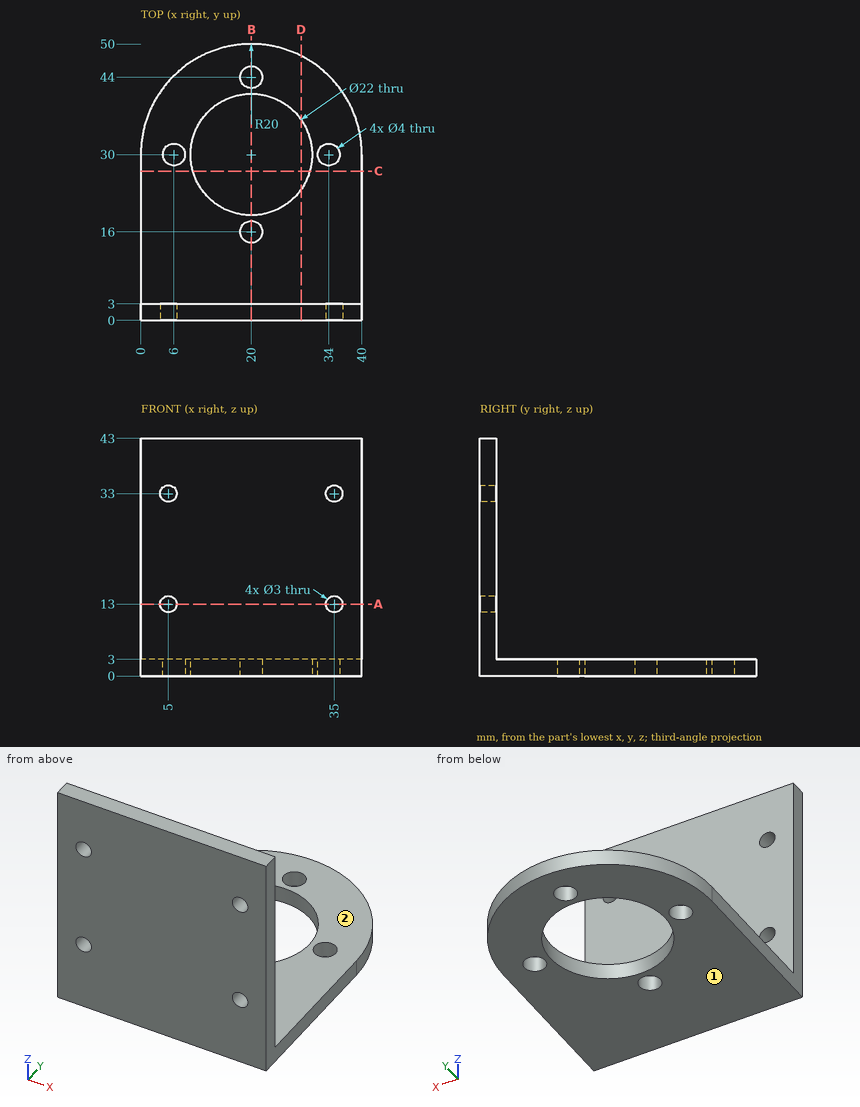
Print and shaded views of the part. All mm, measured from the part's lowest x, y and z. A direction names the side the tool comes from. Coordinates: 2 decimals unless noted, no trailing zeros. Loops run counter-clockwise (first coordinate to the right, second up) from the corner with the lowest first, then second, coordinate; pieces in that order, holes last. Notation, with made-up numbers: (74, -20.75) -> (130, -20.75) arc R24 cw to (130, 10.25) -> close; hole circle Ø11 at (-12.5, 25). An arc over 180 degrees is marked (long way). Use one line per item in the form item = value. Start each with the question number.
(1) Flat gauge pins, fed straight in: pin 1 (10 mm diameter, centred on x = 30, z = 15.5, fed in from +Y); pin 2 (20 mm diameter, centred on x = 25, y = 19.5, fed in from +Z). Where does each tip first touch, or does it go through?
(2) Probe probe 1 along Z at (x, y) = (3.5, 19.5); probe 2 along Y at (x, z) = (34, 2.2). List the from-to ranges inside material, lowest first. Write a range as from..to.
(3) Tool access for the marked faces 1 and 2: list every direction of +Z, -Z, +X, -X, +Y, -Y with a clear straight run to the whole face (end or side of a thin tool).
(4) Cut at A-A on z = 13. Give the cut face in (x, y), and give its area (3 significant figures).
(5) Cut at D-D on x = 29. Give the cut face in (y, z).
(6) Cut at C-C on y = 27. Give the cut face in (x, z).
(7) Cut at B-B on x = 20. Give the cut face in (y, z), and give its area (3 significant figures).
Values:
q1.pin_1 = 3
q1.pin_2 = 3
q2.probe_1 = 0..3
q2.probe_2 = 0..28, 32..44.28
q3.face_1 = -Z, +X, -X, +Y, -Y
q3.face_2 = +Z, +X, -X, +Y
q4.outline = (0, 0) -> (3.5, 0) -> (3.5, 3) -> (0, 3) -> close; (6.5, 0) -> (33.5, 0) -> (33.5, 3) -> (6.5, 3) -> close; (36.5, 0) -> (40, 0) -> (40, 3) -> (36.5, 3) -> close
q4.area = 102 mm2
q5.outline = (0, 0) -> (23.68, 0) -> (23.68, 3) -> (3, 3) -> (3, 43) -> (0, 43) -> close; (36.32, 0) -> (47.86, 0) -> (47.86, 3) -> (36.32, 3) -> close
q6.outline = (0, 0) -> (9.42, 0) -> (9.42, 3) -> (0, 3) -> close; (30.58, 0) -> (40, 0) -> (40, 3) -> (30.58, 3) -> close
q7.outline = (0, 0) -> (14, 0) -> (14, 3) -> (3, 3) -> (3, 43) -> (0, 43) -> close; (18, 0) -> (19, 0) -> (19, 3) -> (18, 3) -> close; (41, 0) -> (42, 0) -> (42, 3) -> (41, 3) -> close; (46, 0) -> (50, 0) -> (50, 3) -> (46, 3) -> close
q7.area = 180 mm2
